Autodesk Inventor part; units mm, degrees
ref_plane "YZ Plane" through (0, 0, 0) normal (1, 0, 0) x (0, 1, 0)
ref_plane "XZ Plane" through (0, 0, 0) normal (0, 1, 0) x (-1, 0, 0)
ref_plane "XY Plane" through (0, 0, 0) normal (0, 0, 1) x (1, 0, 0)
sketch "Sketch1" plane through (0, 0, 0) normal (0, 0, 1) x (1, 0, 0)
  circle A0 centre (0, 0) radius 12.5 construction
  circle A1 centre (0, 8.5) radius 1.5 construction
  circle A2 centre (-7.3612, 4.25) radius 1.5 construction
  circle A3 centre (-7.3612, -4.25) radius 1.5 construction
  circle A4 centre (0, -8.5) radius 1.5 construction
  circle A5 centre (7.3612, -4.25) radius 1.5 construction
  circle A6 centre (7.3612, 4.25) radius 1.5 construction
  circle A7 centre (0, 0) radius 4 construction
  line L0 (45, -12.5) -> (-22.5, -12.5) construction
  line L1 (-22.5, -12.5) -> (-22.5, 12.5) construction
  line L2 (-22.5, 12.5) -> (45, 12.5) construction
  line L3 (45, 12.5) -> (45, -12.5) construction
  line L4 (45, -12.5) -> (-22.5, 12.5) construction
  line L5 (-22.5, -12.5) -> (45, 12.5) construction
  line L6 (-22.5, -12.5) -> (-12.5, -12.5) construction
  line L7 (-12.5, -12.5) -> (-12.5, -15.5) construction
  line L8 (-12.5, -15.5) -> (-22.5, -15.5) construction
  line L9 (-22.5, -15.5) -> (-22.5, -12.5) construction
  line L10 (12.5, -12.5) -> (22.5, -12.5) construction
  line L11 (22.5, -12.5) -> (22.5, -15.5) construction
  line L12 (22.5, -15.5) -> (12.5, -15.5) construction
  line L13 (12.5, -15.5) -> (12.5, -12.5) construction
  line L14 (-22.5, 12.5) -> (-12.5, 12.5) construction
  line L15 (-12.5, 12.5) -> (-12.5, 15.5) construction
  line L16 (-12.5, 15.5) -> (-22.5, 15.5) construction
  line L17 (-22.5, 15.5) -> (-22.5, 12.5) construction
  line L18 (12.5, 12.5) -> (22.5, 12.5) construction
  line L19 (22.5, 12.5) -> (22.5, 15.5) construction
  line L20 (22.5, 15.5) -> (12.5, 15.5) construction
  line L21 (12.5, 15.5) -> (12.5, 12.5) construction
  line L22 (45, 12.5) -> (42, 12.5) construction
  line L23 (42, 12.5) -> (42, 7.5) construction
  line L24 (42, 7.5) -> (45, 7.5) construction
  line L25 (45, 7.5) -> (45, 12.5) construction
  line L26 (45, -12.5) -> (42, -12.5) construction
  line L27 (42, -12.5) -> (42, -7.5) construction
  line L28 (42, -7.5) -> (45, -7.5) construction
  line L29 (45, -7.5) -> (45, -12.5) construction
  point P0 (11.25, 0)
  dimension "d0" = 25
  dimension "d1" = 3
  dimension "d2" = 8.5
  dimension "d5" = 360
  dimension "d7" = 8
  dimension "d8" = 10
  dimension "d9" = 3
  dimension "d10" = 10
  dimension "d11" = 3
  dimension "d12" = 22.5
  dimension "d13" = 10
  dimension "d14" = 3
  dimension "d15" = 10
  dimension "d16" = 3
  dimension "d17" = 3
  dimension "d18" = 5
  dimension "d19" = 3
  dimension "d20" = 5
sketch "Sketch2" plane through (0, 0, 0) normal (0, 0, 1) x (1, 0, 0)
  line L0 (45, -12.5) -> (-22.5, -12.5) construction
  line L1 (-22.5, -12.5) -> (-22.5, 12.5) construction
  line L2 (-22.5, 12.5) -> (45, 12.5) construction
  line L3 (-22.5, 12.5) -> (45, 12.5)
  line L4 (45, 12.5) -> (45, -12.5)
  line L5 (45, -12.5) -> (-22.5, -12.5)
  line L6 (-22.5, -12.5) -> (-22.5, 12.5)
  point P0 (0, 0)
extrude "Extrusion1" add sketch "Sketch2" along normal blind 3
sketch "Sketch3" plane through (0, 0, 0) normal (0, 0, -1) x (-1, 0, 0)
  line L0 (12.5, 15.5) -> (22.5, 15.5) construction
  line L1 (12.5, 12.5) -> (12.5, 15.5) construction
  line L2 (22.5, 12.5) -> (12.5, 12.5)
  line L3 (12.5, 12.5) -> (12.5, 15.5)
  line L4 (12.5, 15.5) -> (22.5, 15.5)
  line L5 (22.5, 15.5) -> (22.5, 12.5)
  line L6 (-22.5, 15.5) -> (-12.5, 15.5) construction
  line L7 (-22.5, 12.5) -> (-22.5, 15.5) construction
  line L8 (-12.5, 15.5) -> (-12.5, 12.5) construction
  line L9 (-12.5, 12.5) -> (-22.5, 12.5)
  line L10 (-22.5, 12.5) -> (-22.5, 15.5)
  line L11 (-22.5, 15.5) -> (-12.5, 15.5)
  line L12 (-12.5, 15.5) -> (-12.5, 12.5)
  point P0 (0, 0)
extrude "Extrusion2" add sketch "Sketch3" against normal blind 3
sketch "Sketch4" plane through (0, 0, 0) normal (0, 0, -1) x (-1, 0, 0)
  line L0 (-42, 12.5) -> (-42, 7.5) construction
  line L1 (-42, 7.5) -> (-45, 7.5) construction
  line L2 (-45, 12.5) -> (-42, 12.5)
  line L3 (-42, 12.5) -> (-42, 7.5)
  line L4 (-42, 7.5) -> (-45, 7.5)
  line L5 (-45, 7.5) -> (-45, 12.5)
  point P0 (0, 0)
extrude "Extrusion3" cut sketch "Sketch4" against normal blind 3
sketch "Sketch5" plane through (0, 0, 0) normal (0, 0, -1) x (-1, 0, 0)
  circle A0 centre (0, 0) radius 4 construction
  circle A1 centre (0, 8.5) radius 1.5 construction
  circle A2 centre (0, 0) radius 4
extrude "Extrusion4" cut sketch "Sketch5" against normal blind 3
sketch "Sketch6" plane through (0, 0, 0) normal (0, 0, -1) x (-1, 0, 0)
  circle A0 centre (0, 8.5) radius 1.5 construction
  circle A1 centre (0, 8.5) radius 1.5
  point P0 (0, 0)
extrude "Extrusion5" cut sketch "Sketch6" against normal blind 3
mirror "Mirror1" about plane through (0, 0, 0) normal (0, 1, 0) of "Extrusion2", "Extrusion3"
pattern_circular "Circular Pattern1" count 6 over 360 about axis through (0, 0, 0) along (0, 0, 1) of "Extrusion5"
sketch "Sketch7" plane through (0, 0, 0) normal (0, 0, -1) x (-1, 0, 0)
  line L0 (12.5, 5) -> (15.5, 5)
  line L1 (15.5, 5) -> (15.5, -5)
  line L2 (15.5, -5) -> (12.5, -5)
  line L3 (12.5, -5) -> (12.5, 5)
  line L4 (12.5, 15.5) -> (12.5, 12.5)
  line L5 (22.5, -15.5) -> (22.5, 15.5)
  line L6 (-12.5, 5) -> (-15.5, 5)
  line L7 (-15.5, 5) -> (-15.5, -5)
  line L8 (-15.5, -5) -> (-12.5, -5)
  line L9 (-12.5, -5) -> (-12.5, 5)
  line L10 (-12.5, 12.5) -> (-12.5, 15.5)
  point P0 (0, 0)
  point P1 (15.5, 0)
  point P2 (22.5, 0)
  dimension "d34" = 3
  dimension "d35" = 10
  dimension "d36" = 3
  dimension "d37" = 10
extrude "Extrusion6" cut sketch "Sketch7" against normal blind 3
properties part number "Motor mount"
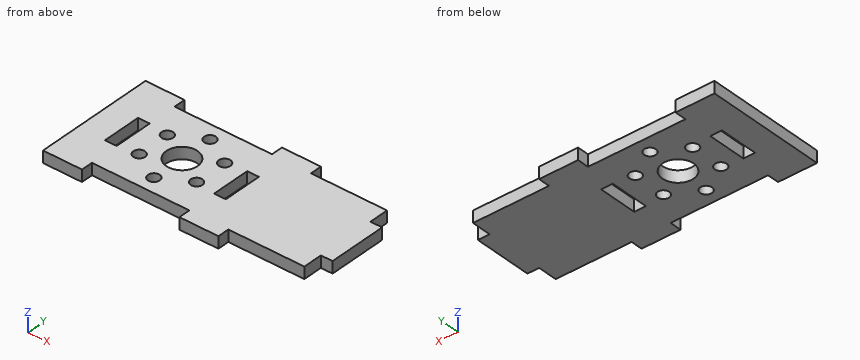
Part model, mm, in its own coordinate system. Round coordinates to 2 decimals unless told otherwise and drop trailing zeros. Loops run counter-clockwise (first coordinate to the right, second up) from the corner with the lowest first, then second, coordinate; pieces in that order, holes last. Notation, with made-up numbers: (40, 1.25) -> (59, 1.25) arc R19 ccw to (59, 33.25) -> close; hole circle Ø7 at (75.25, 28). An arc over 180 degrees is marked (long way). Use a Markdown table: item, result.
1) Drop flat-ended pins along their axis: pin 1 Ø8 at (x, y) = (6.5, 6.5) entering from -Z; pin 2 Ø1.5 at (y, z) = (13.5, 1.5) entering from +X; pin 3 Ø0.9 at (y, z) = (-10.5, 1.5) entering from +X; pin 4 Ø2.5 at (x, y) = (7.36, 4.25) entering from -Z. Give the stop position or say it passes through.
The answers:
| item | result |
|---|---|
| pin 1 | stops at z = 0 |
| pin 2 | stops at x = 22.5 |
| pin 3 | stops at x = 42 |
| pin 4 | passes through |
2) Cut at A-A, the plane y = -8.5. List the corners of the cut face in (x, z), and give its area (4 significant figures).
The answers:
| item | result |
|---|---|
| outline | (-22.5, 0) -> (-1.5, 0) -> (-1.5, 3) -> (-22.5, 3) -> close; (1.5, 0) -> (42, 0) -> (42, 3) -> (1.5, 3) -> close |
| area | 184.5 mm2 |
3) Cut at C-C, the plane y = 2. List the corners of the cut face in (x, z).
The answers:
| item | result |
|---|---|
| outline | (-22.5, 0) -> (-15.5, 0) -> (-15.5, 3) -> (-22.5, 3) -> close; (-12.5, 0) -> (-3.46, 0) -> (-3.46, 3) -> (-12.5, 3) -> close; (3.46, 0) -> (12.5, 0) -> (12.5, 3) -> (3.46, 3) -> close; (15.5, 0) -> (45, 0) -> (45, 3) -> (15.5, 3) -> close |
4) Cut at D-D, the plane z = 0.8. State how many separate pieces and enclosed holes the cut face has, and give its area (3 significant figures).
The answers:
| item | result |
|---|---|
| separate pieces | 1 |
| enclosed holes | 9 |
| area | 1,620 mm2 |
5) Probe line 1 (Y direction, x = 0, z = 0.75); line 2 (Y direction, x = 11.5, z = 1.75); line 3 (X direction, y = 11, z = 1.9). List the from-to ranges inside material, lowest first. Write a range as [from, to].
The answers:
| item | result |
|---|---|
| line 1 | y = [-12.5, -10], [-7, -4], [4, 7], [10, 12.5] |
| line 2 | y = [-12.5, 12.5] |
| line 3 | x = [-22.5, 42] |
6) Cut at B-B, the plane x = 0. List the corners of the cut face in (y, z).
The answers:
| item | result |
|---|---|
| outline | (-12.5, 0) -> (-10, 0) -> (-10, 3) -> (-12.5, 3) -> close; (-7, 0) -> (-4, 0) -> (-4, 3) -> (-7, 3) -> close; (4, 0) -> (7, 0) -> (7, 3) -> (4, 3) -> close; (10, 0) -> (12.5, 0) -> (12.5, 3) -> (10, 3) -> close |
